Work out the finished part from the listing and answer in its coordinate system (mm). A direction names the side the tool comes from. Round coordinates to 2 decimals unless told otherwise and drop trailing zeros. Loops run counter-clockwise (first coordinate to the right, second up) from the corner with the lowest first, then second, coordinate; pieces in that order, holes last. Notation, with made-up numbers: (0.25, -32) - (48.25, -32) arc R20 cw to (48.25, -20) - close; hole circle Ø9 at (9, -36.5). An arc over 180 degrees is marked (long way). Return JSON: item names as keys, results as strings.
from build123d import *

# Parameters (mm, degrees)
SKETCH_1_W          = 112
SKETCH_1_H          = 58
EXTRUDE_1_DEPTH     = 4
SKETCH_2_OUTSIDE_W  = 139.238
SKETCH_2_OUTSIDE_H  = 85.238
CUT_EXTRUDE_1_DEPTH = 4
SKETCH_3_R          = 11.25
CUT_EXTRUDE_2_DEPTH = 4
CUT_EXTRUDE_3_REACH = 65.19
SKETCH_4_R          = 1.65
SKETCH_4_R_2        = 1.7
CUT_EXTRUDE_4_REACH = 65.19
SKETCH_5_R          = 1.25
SKETCH_8_W          = 6
SKETCH_8_H          = 30
EXTRUDE_3_DEPTH     = 4
CUT_EXTRUDE_5_REACH = 70.564
SKETCH_10_R         = 1.65
CUT_EXTRUDE_6_REACH = 70.564
SKETCH_11_R         = 1.65
SKETCH_13_R         = 1.4
CUT_EXTRUDE_7_DEPTH = 69.563838866


with BuildPart() as part:
    # 草图1 → 凸台-拉伸1 (new body)
    with BuildSketch(Plane.XY):
        Rectangle(SKETCH_1_W, SKETCH_1_H)
    extrude(amount=EXTRUDE_1_DEPTH)

    # 草图2 outside → 切除-拉伸1 (cut)
    with BuildSketch(Plane.XY.offset(4)):
        Rectangle(SKETCH_2_OUTSIDE_W, SKETCH_2_OUTSIDE_H)
        Polygon((56, 1), (-14, 1), (-28, 15), (-28, 29), (-56, 29), (-56, 1), (-26, -29), (56, -29), align=None, mode=Mode.SUBTRACT)
    extrude(amount=-CUT_EXTRUDE_1_DEPTH, mode=Mode.SUBTRACT)

    # 草图3 → 切除-拉伸2 (cut)
    with BuildSketch(Plane.XY.offset(4)):
        with Locations((-42, 15)):
            Circle(SKETCH_3_R)
    extrude(amount=-CUT_EXTRUDE_2_DEPTH, mode=Mode.SUBTRACT)

    # 草图4 → 切除-拉伸3 (cut, up to next)
    with BuildSketch(Plane.XY.offset(4), mode=Mode.PRIVATE) as cut_extrude_3_sk1:
        with Locations((-22.5, -19)):
            Circle(SKETCH_4_R)
    cut_extrude_3_tool1 = extrude(cut_extrude_3_sk1.sketch, amount=-CUT_EXTRUDE_3_REACH, mode=Mode.PRIVATE) & part.part
    # 草图4 → 切除-拉伸3 (cut, up to next)
    with BuildSketch(Plane.XY.offset(4), mode=Mode.PRIVATE) as cut_extrude_3_sk2:
        with Locations((-22.5, -9)):
            Circle(SKETCH_4_R)
    cut_extrude_3_tool2 = extrude(cut_extrude_3_sk2.sketch, amount=-CUT_EXTRUDE_3_REACH, mode=Mode.PRIVATE) & part.part
    # 草图4 → 切除-拉伸3 (cut, up to next)
    with BuildSketch(Plane.XY.offset(4), mode=Mode.PRIVATE) as cut_extrude_3_sk3:
        with Locations((-7.5, -19)):
            Circle(SKETCH_4_R)
    cut_extrude_3_tool3 = extrude(cut_extrude_3_sk3.sketch, amount=-CUT_EXTRUDE_3_REACH, mode=Mode.PRIVATE) & part.part
    # 草图4 → 切除-拉伸3 (cut, up to next)
    with BuildSketch(Plane.XY.offset(4), mode=Mode.PRIVATE) as cut_extrude_3_sk4:
        with Locations((-7.5, -9)):
            Circle(SKETCH_4_R)
    cut_extrude_3_tool4 = extrude(cut_extrude_3_sk4.sketch, amount=-CUT_EXTRUDE_3_REACH, mode=Mode.PRIVATE) & part.part
    # 草图4 → 切除-拉伸3 (cut, up to next)
    with BuildSketch(Plane.XY.offset(4), mode=Mode.PRIVATE) as cut_extrude_3_sk5:
        with Locations((38.5, -19)):
            Circle(SKETCH_4_R)
    cut_extrude_3_tool5 = extrude(cut_extrude_3_sk5.sketch, amount=-CUT_EXTRUDE_3_REACH, mode=Mode.PRIVATE) & part.part
    # 草图4 → 切除-拉伸3 (cut, up to next)
    with BuildSketch(Plane.XY.offset(4), mode=Mode.PRIVATE) as cut_extrude_3_sk6:
        with Locations((38.5, -9)):
            Circle(SKETCH_4_R)
    cut_extrude_3_tool6 = extrude(cut_extrude_3_sk6.sketch, amount=-CUT_EXTRUDE_3_REACH, mode=Mode.PRIVATE) & part.part
    # 草图4 → 切除-拉伸3 (cut, up to next)
    with BuildSketch(Plane.XY.offset(4), mode=Mode.PRIVATE) as cut_extrude_3_sk7:
        with Locations((53.5, -19)):
            Circle(SKETCH_4_R)
    cut_extrude_3_tool7 = extrude(cut_extrude_3_sk7.sketch, amount=-CUT_EXTRUDE_3_REACH, mode=Mode.PRIVATE) & part.part
    # 草图4 → 切除-拉伸3 (cut, up to next)
    with BuildSketch(Plane.XY.offset(4), mode=Mode.PRIVATE) as cut_extrude_3_sk8:
        with Locations((53.5, -9)):
            Circle(SKETCH_4_R)
    cut_extrude_3_tool8 = extrude(cut_extrude_3_sk8.sketch, amount=-CUT_EXTRUDE_3_REACH, mode=Mode.PRIVATE) & part.part
    # 草图4 → 切除-拉伸3 (cut, up to next)
    with BuildSketch(Plane.XY.offset(4), mode=Mode.PRIVATE) as cut_extrude_3_sk9:
        with Locations((19, -25)):
            Circle(SKETCH_4_R_2)
    cut_extrude_3_tool9 = extrude(cut_extrude_3_sk9.sketch, amount=-CUT_EXTRUDE_3_REACH, mode=Mode.PRIVATE) & part.part
    # 草图4 → 切除-拉伸3 (cut, up to next)
    with BuildSketch(Plane.XY.offset(4), mode=Mode.PRIVATE) as cut_extrude_3_sk10:
        with Locations((29, -25)):
            Circle(SKETCH_4_R_2)
    cut_extrude_3_tool10 = extrude(cut_extrude_3_sk10.sketch, amount=-CUT_EXTRUDE_3_REACH, mode=Mode.PRIVATE) & part.part
    add(cut_extrude_3_tool1.solids().sort_by_distance((-22.5, -19, 4))[0], mode=Mode.SUBTRACT)
    add(cut_extrude_3_tool2.solids().sort_by_distance((-22.5, -9, 4))[0], mode=Mode.SUBTRACT)
    add(cut_extrude_3_tool3.solids().sort_by_distance((-7.5, -19, 4))[0], mode=Mode.SUBTRACT)
    add(cut_extrude_3_tool4.solids().sort_by_distance((-7.5, -9, 4))[0], mode=Mode.SUBTRACT)
    add(cut_extrude_3_tool5.solids().sort_by_distance((38.5, -19, 4))[0], mode=Mode.SUBTRACT)
    add(cut_extrude_3_tool6.solids().sort_by_distance((38.5, -9, 4))[0], mode=Mode.SUBTRACT)
    add(cut_extrude_3_tool7.solids().sort_by_distance((53.5, -19, 4))[0], mode=Mode.SUBTRACT)
    add(cut_extrude_3_tool8.solids().sort_by_distance((53.5, -9, 4))[0], mode=Mode.SUBTRACT)
    add(cut_extrude_3_tool9.solids().sort_by_distance((19, -25, 4))[0], mode=Mode.SUBTRACT)
    add(cut_extrude_3_tool10.solids().sort_by_distance((29, -25, 4))[0], mode=Mode.SUBTRACT)

    # 草图5 → 切除-拉伸4 (cut, up to next)
    with BuildSketch(Plane(origin=(0, 0, 0), x_dir=(-1, 0, 0), z_dir=(0, 0, -1)), mode=Mode.PRIVATE) as cut_extrude_4_sk1:
        with Locations((-16.406007896, -13.5)):
            Circle(SKETCH_5_R)
    cut_extrude_4_tool1 = extrude(cut_extrude_4_sk1.sketch, amount=-CUT_EXTRUDE_4_REACH, mode=Mode.PRIVATE) & part.part
    # 草图5 → 切除-拉伸4 (cut, up to next)
    with BuildSketch(Plane(origin=(0, 0, 0), x_dir=(-1, 0, 0), z_dir=(0, 0, -1)), mode=Mode.PRIVATE) as cut_extrude_4_sk2:
        with Locations((-24.406007896, -13.5)):
            Circle(SKETCH_5_R)
    cut_extrude_4_tool2 = extrude(cut_extrude_4_sk2.sketch, amount=-CUT_EXTRUDE_4_REACH, mode=Mode.PRIVATE) & part.part
    # 草图5 → 切除-拉伸4 (cut, up to next)
    with BuildSketch(Plane(origin=(0, 0, 0), x_dir=(-1, 0, 0), z_dir=(0, 0, -1)), mode=Mode.PRIVATE) as cut_extrude_4_sk3:
        with Locations((-16.406007896, -1.5)):
            Circle(SKETCH_5_R)
    cut_extrude_4_tool3 = extrude(cut_extrude_4_sk3.sketch, amount=-CUT_EXTRUDE_4_REACH, mode=Mode.PRIVATE) & part.part
    # 草图5 → 切除-拉伸4 (cut, up to next)
    with BuildSketch(Plane(origin=(0, 0, 0), x_dir=(-1, 0, 0), z_dir=(0, 0, -1)), mode=Mode.PRIVATE) as cut_extrude_4_sk4:
        with Locations((-24.406007896, -1.5)):
            Circle(SKETCH_5_R)
    cut_extrude_4_tool4 = extrude(cut_extrude_4_sk4.sketch, amount=-CUT_EXTRUDE_4_REACH, mode=Mode.PRIVATE) & part.part
    # 草图5 → 切除-拉伸4 (cut, up to next)
    with BuildSketch(Plane(origin=(0, 0, 0), x_dir=(-1, 0, 0), z_dir=(0, 0, -1)), mode=Mode.PRIVATE) as cut_extrude_4_sk5:
        with Locations((31.779946847, -13.5)):
            Circle(SKETCH_5_R)
    cut_extrude_4_tool5 = extrude(cut_extrude_4_sk5.sketch, amount=-CUT_EXTRUDE_4_REACH, mode=Mode.PRIVATE) & part.part
    # 草图5 → 切除-拉伸4 (cut, up to next)
    with BuildSketch(Plane(origin=(0, 0, 0), x_dir=(-1, 0, 0), z_dir=(0, 0, -1)), mode=Mode.PRIVATE) as cut_extrude_4_sk6:
        with Locations((31.779946847, -1.5)):
            Circle(SKETCH_5_R)
    cut_extrude_4_tool6 = extrude(cut_extrude_4_sk6.sketch, amount=-CUT_EXTRUDE_4_REACH, mode=Mode.PRIVATE) & part.part
    add(cut_extrude_4_tool1.solids().sort_by_distance((16.406008, -13.5, 0))[0], mode=Mode.SUBTRACT)
    add(cut_extrude_4_tool2.solids().sort_by_distance((24.406008, -13.5, 0))[0], mode=Mode.SUBTRACT)
    add(cut_extrude_4_tool3.solids().sort_by_distance((16.406008, -1.5, 0))[0], mode=Mode.SUBTRACT)
    add(cut_extrude_4_tool4.solids().sort_by_distance((24.406008, -1.5, 0))[0], mode=Mode.SUBTRACT)
    add(cut_extrude_4_tool5.solids().sort_by_distance((-31.779947, -13.5, 0))[0], mode=Mode.SUBTRACT)
    add(cut_extrude_4_tool6.solids().sort_by_distance((-31.779947, -1.5, 0))[0], mode=Mode.SUBTRACT)

    # 草图8 → 凸台-拉伸3 (add)
    with BuildSketch(Plane(origin=(0, 0, 0), x_dir=(-1, 0, 0), z_dir=(0, 0, -1))):
        with Locations((-59, -14)):
            Rectangle(SKETCH_8_W, SKETCH_8_H)
    extrude(amount=-EXTRUDE_3_DEPTH)

    # 草图10 → 切除-拉伸5 (cut, up to next)
    with BuildSketch(Plane.XY.offset(4), mode=Mode.PRIVATE) as cut_extrude_5_sk1:
        with Locations((59, -25)):
            Circle(SKETCH_10_R)
    cut_extrude_5_tool1 = extrude(cut_extrude_5_sk1.sketch, amount=-CUT_EXTRUDE_5_REACH, mode=Mode.PRIVATE) & part.part
    # 草图10 → 切除-拉伸5 (cut, up to next)
    with BuildSketch(Plane.XY.offset(4), mode=Mode.PRIVATE) as cut_extrude_5_sk2:
        with Locations((59, -3)):
            Circle(SKETCH_10_R)
    cut_extrude_5_tool2 = extrude(cut_extrude_5_sk2.sketch, amount=-CUT_EXTRUDE_5_REACH, mode=Mode.PRIVATE) & part.part
    add(cut_extrude_5_tool1.solids().sort_by_distance((59, -25, 4))[0], mode=Mode.SUBTRACT)
    add(cut_extrude_5_tool2.solids().sort_by_distance((59, -3, 4))[0], mode=Mode.SUBTRACT)

    # 草图11 → 切除-拉伸6 (cut, up to next)
    with BuildSketch(Plane.XY.offset(4), mode=Mode.PRIVATE) as cut_extrude_6_sk1:
        with Locations((-28.036589911, -20.593670707)):
            Circle(SKETCH_11_R)
    cut_extrude_6_tool1 = extrude(cut_extrude_6_sk1.sketch, amount=-CUT_EXTRUDE_6_REACH, mode=Mode.PRIVATE) & part.part
    add(cut_extrude_6_tool1.solids().sort_by_distance((-28.03659, -20.593671, 4))[0], mode=Mode.SUBTRACT)

    # 草图13 → 切除-拉伸7 (cut, through all)
    with BuildSketch(Plane(origin=(0, 0, 0), x_dir=(-1, 0, 0), z_dir=(0, 0, -1))):
        with Locations((53.5, 26.5)):
            Circle(SKETCH_13_R)
        with Locations((53.5, 3.5)):
            Circle(SKETCH_13_R)
        with Locations((30.5, 3.5)):
            Circle(SKETCH_13_R)
        with Locations((30.5, 26.5)):
            Circle(SKETCH_13_R)
    extrude(amount=-CUT_EXTRUDE_7_DEPTH, mode=Mode.SUBTRACT)


solid = part.part
1) Section C-C (y = 16.5) is taken. Give the vertices of the cut face in (x, z), and give its area (3 significant figures).
Verdict:
{"outline": "(-56, 0) - (-53.15, 0) - (-53.15, 4) - (-56, 4) - close; (-30.85, 0) - (-28, 0) - (-28, 4) - (-30.85, 4) - close", "area": "22.8 mm2"}
2) Determine the mould class of faces 3 (the cylindrical face through (51.85, -18.93, 2.03)), 4 (the flat face through (-21, 8, 2)), 5 (the flat face through (4, -6, 0)) for opening direction X: pulls with the +X half, pulls with the -X half, needs draft (parallel to the pull), parting line crosses it, or undercut.
Verdict:
{"face 3": "undercut", "face 4": "pulls with the +X half", "face 5": "needs draft"}
3) Section B-B (x = -22.5) is taken. Give the vertices of the cut face in (y, z), and give its area (3 significant figures).
Verdict:
{"outline": "(-29, 0) - (-20.65, 0) - (-20.65, 4) - (-29, 4) - close; (-17.35, 0) - (-10.65, 0) - (-10.65, 4) - (-17.35, 4) - close; (-7.35, 0) - (9.5, 0) - (9.5, 4) - (-7.35, 4) - close", "area": "128 mm2"}
4) Flat-ended cylindrical pins translate along their axes: pin 1 (12 mm diameter, centred on x = 2, y = -18, fed in from -Z); pin 2 (2 mm diameter, centred on y = 7, z = 3, fed in from +X); pin 3 (2 mm diameter, centred on x = -31.78, y = -1.5, fed in from +Z); pin 4 (1.5 mm diameter, centred on x = 29.5, z = 3, fed in from +Y). Find the tip coordinate at first contact, or state that the pin passes through.
Verdict:
{"pin 1": "stops at z = 0", "pin 2": "stops at x = -19", "pin 3": "passes through", "pin 4": "stops at y = 1"}
5) Find the intervals of material crossed by L1, parallel to Y at x = -7.5, z = 2.1; L2, parallel to X at y = -19.5, z = 0.6; L3, parallel to Y at x = 51, z = 2.3, in increasing order.
Verdict:
{"L1": "y = -29 to -20.65, -17.35 to -10.65, -7.35 to 1", "L2": "x = -35.5 to -29.27, -26.8 to -24.07, -20.93 to -9.07, -5.93 to 36.93, 40.07 to 51.93, 55.07 to 62", "L3": "y = -29 to 1"}
6) Section D-D (z = 2.85) is taken. Count the separate pieces of the cut face and the enclosed holes in it, and give its area (3 significant figures).
Verdict:
{"separate pieces": "1", "enclosed holes": "24", "area": "3,410 mm2"}
7) Section A-A (y = -25) is taken. Give the vertices of the cut face in (x, z), and give its area (3 significant figures).
Verdict:
{"outline": "(-30, 0) - (17.3, 0) - (17.3, 4) - (-30, 4) - close; (20.7, 0) - (27.3, 0) - (27.3, 4) - (20.7, 4) - close; (30.7, 0) - (57.35, 0) - (57.35, 4) - (30.7, 4) - close; (60.65, 0) - (62, 0) - (62, 4) - (60.65, 4) - close", "area": "328 mm2"}
8) A tool of negligible diameter and unlimited length cuts with its end or side. For faces 1 (the flat face through (25, 1, 2)), 2 (the cylindrical face through (-50.928, 8.155, 2.028)), from which of +Z, -Z, +X, -X, +Y, -Y can it reach the whole face along a straight path? Write none if from no direction.
Verdict:
{"face 1": "+Z, -Z, +X, +Y", "face 2": "+Z, -Z"}
